Job drawing, mm, ordinate dimensions from the low corner. One solid piece. Give positions to 0.01 mm unless a question says otherwise; leave off trailing zeros. Write each loop counter-clockwise with the first axis right and the second up, starting at its lowest first coordinate (ties: lowest second). Pieces come first, ordered by that corner, then holes. Notation, with made-up numbers: (18, 33.5) - (34, 33.5) arc R4 ccw to (34, 39.5) - close; hole circle Ø9 at (17, 78). An arc over 180 degrees is marked (long way). Answer as a JSON object with one key per item and string values.
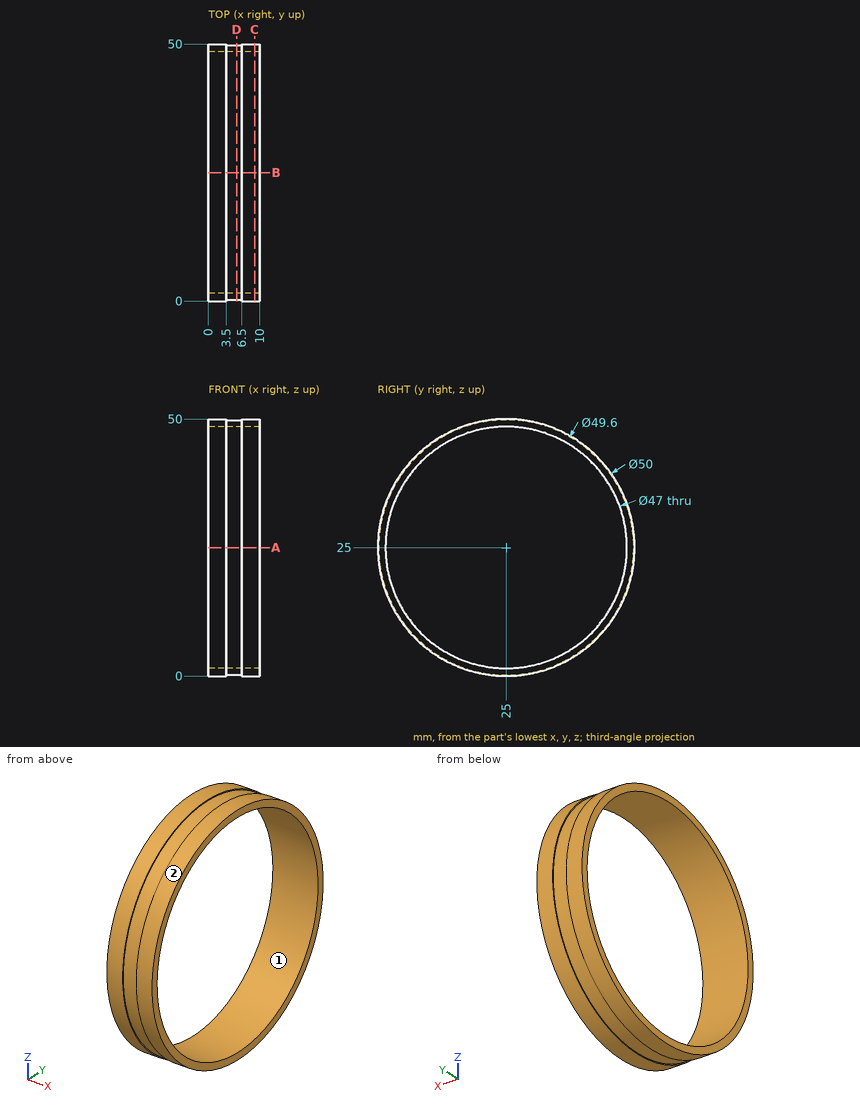
Item 1: Mould opens along Y. For the marked faces 1 and 2 say: +Y half, -Y half, draft (parallel to the pull), parting line (faces both ways), or undercut.
Entries:
{"face 1": "undercut", "face 2": "parting line"}
Item 2: Probe line 1 (Y direction, x = 7.25, z = 25); line 2 (Y direction, x = 5, z = 25). List the from-to ranges inside material, lowest first. Write a range as from..to.
Entries:
{"line 1": "0..1.5, 48.5..50", "line 2": "0.2..1.5, 48.5..49.8"}
Item 3: Cut at C-C (x = 9). Give the cut face in (y, z).
Entries:
{"outline": "circle Ø50 at (25, 25); hole circle Ø47 at (25, 25)"}
Item 4: Cut at A-A (z = 25). Give the cut face in (x, y).
Entries:
{"outline": "(0, 0) - (3.5, 0) - (3.5, 0.2) - (6.5, 0.2) - (6.5, 0) - (10, 0) - (10, 1.5) - (0, 1.5) - close; (0, 48.5) - (10, 48.5) - (10, 50) - (6.5, 50) - (6.5, 49.8) - (3.5, 49.8) - (3.5, 50) - (0, 50) - close"}
Item 5: Flat gauge pins, fed straight in: P1, Ø3, axis at x = 4, z = 36, coming from the -Y side; P2, Ø2, axis at x = 8.5, z = 40, coming from the -Y side; P3, Ø1.5, axis at x = 1.5, z = 32.5, coming from the -Y side. Where does each tip first touch, or does it go through?
Entries:
{"P1": "y = 1.91", "P2": "y = 4.29", "P3": "y = 0.93"}
Item 6: Cut at D-D (x = 5.5). Give the cut face in (y, z).
Entries:
{"outline": "circle Ø49.6 at (25, 25); hole circle Ø47 at (25, 25)"}
